```python
from build123d import *

# Parameters (mm, degrees)
SKETCH_1_W          = 210
SKETCH_1_H          = 100
EXTRUDE_1_DEPTH     = 5
FILLET_1_R          = 5
SKETCH_2_R          = 1.5
CUT_EXTRUDE_1_DEPTH = 5
SKETCH_4_R          = 2.25
CUT_EXTRUDE_2_DEPTH = 5
SKETCH_6_R          = 1.5
CUT_EXTRUDE_3_DEPTH = 5


with BuildPart() as part:
    # 草图1 → 凸台-拉伸1 (new body)
    with BuildSketch(Plane(origin=(0, 0, 0), x_dir=(1, 0, 0), z_dir=(0, 1, 0))):
        with Locations((-105, 50)):
            Rectangle(SKETCH_1_W, SKETCH_1_H)
    extrude(amount=EXTRUDE_1_DEPTH)

    # 圆角1
    fillet_1_edges = [part.edges().sort_by_distance(p)[0] for p in [
        (-210, 2.5, -100),
        (0, 2.5, -100),
        (0, 2.5, 0),
        (-210, 2.5, 0),
    ]]
    fillet(fillet_1_edges, radius=FILLET_1_R)

    # 草图2 → 切除-拉伸1 (cut)
    with BuildSketch(Plane(origin=(0, 5, 0), x_dir=(1, 0, 0), z_dir=(0, 1, 0))):
        with Locations(Location((-205, 90, 0), (0, 0, 270))):
            Circle(SKETCH_2_R)
        with Locations(Location((-205, 10, 0), (0, 0, 270))):
            Circle(SKETCH_2_R)
        with Locations(Location((-5, 10, 0), (0, 0, 270))):
            Circle(SKETCH_2_R)
        with Locations(Location((-5, 90, 0), (0, 0, 270))):
            Circle(SKETCH_2_R)
    extrude(amount=-CUT_EXTRUDE_1_DEPTH, mode=Mode.SUBTRACT)

    # 草图4 → 切除-拉伸2 (cut)
    with BuildSketch(Plane.XZ):
        with Locations(Location((-119.1, -45, 0), (0, 0, 270))):
            Circle(SKETCH_4_R)
        with Locations(Location((-119.1, -55, 0), (0, 0, 90))):
            Circle(SKETCH_4_R)
        with Locations(Location((-71.1, -55, 0), (0, 0, 270))):
            Circle(SKETCH_4_R)
        with Locations(Location((-71.1, -45, 0), (0, 0, 90))):
            Circle(SKETCH_4_R)
        Polygon((-115.1, -60), (-75.1, -60), (-75.1, -51), (-71.1, -51), (-71.1, -49), (-75.1, -49), (-75.1, -40), (-115.1, -40), (-115.1, -49), (-119.1, -49), (-119.1, -51), (-115.1, -51), align=None)
    extrude(amount=-CUT_EXTRUDE_2_DEPTH, mode=Mode.SUBTRACT)

    # 草图6 → 切除-拉伸3 (cut)
    with BuildSketch(Plane.XZ):
        with Locations(Location((-40, -41, 0), (0, 0, 270))):
            Circle(SKETCH_6_R)
        with Locations(Location((-40, -59, 0), (0, 0, 270))):
            Circle(SKETCH_6_R)
        with Locations(Location((-170, -59, 0), (0, 0, 90))):
            Circle(SKETCH_6_R)
        with Locations(Location((-170, -41, 0), (0, 0, 90))):
            Circle(SKETCH_6_R)
        with Locations(Location((-185.5, -87, 0), (0, 0, 270))):
            Circle(SKETCH_6_R)
        with Locations(Location((-185.5, -61, 0), (0, 0, 270))):
            Circle(SKETCH_6_R)
        with Locations(Location((-154.5, -87, 0), (0, 0, 90))):
            Circle(SKETCH_6_R)
        with Locations(Location((-154.5, -61, 0), (0, 0, 90))):
            Circle(SKETCH_6_R)
        with Locations(Location((-55.5, -87, 0), (0, 0, 270))):
            Circle(SKETCH_6_R)
        with Locations(Location((-24.5, -87, 0), (0, 0, 90))):
            Circle(SKETCH_6_R)
        with Locations(Location((-55.5, -61, 0), (0, 0, 270))):
            Circle(SKETCH_6_R)
        with Locations(Location((-24.5, -61, 0), (0, 0, 90))):
            Circle(SKETCH_6_R)
    extrude(amount=-CUT_EXTRUDE_3_DEPTH, mode=Mode.SUBTRACT)


solid = part.part
```
CAD build for the part. Positions are in the model's coordinates, mm. A direction names the side the tool comes from. Coordinates: 2 decimals unless noted, no trailing zeros. Write each loop counter-clockwise with the first axis right and the second up, starting at its lowest first coordinate (ties: lowest second). Pieces come first, ordered by that corner, then holes. Notation, with made-up numbers: (-36.5, -30.75) -> (-5.5, -30.75) arc R31 ccw to (-5.5, 2.25) -> close; hole circle Ø4 at (47, 69). An arc over 180 degrees is marked (long way). Return JSON: item names as keys, results as strings. Group by question number.
Q1. Cut at C-C, the plane y = 2.8. State how many separate pieces and enclosed holes the cut face has, then the cut area to 3 significant figures.
Q2. Pull direction Z, two halves, no side cores. Call faces 1 (the face through (-121.296, 2.465, -44.512)), 2 (the face through (-71.001, 2.465, -52.752)), 3 (the face through (-106, 0, -62)), 4 (the face through (-209, 3, -2)): released by +Z, released by -Z, zero draft, split by the parting line, or undercut.
Q3. Cut at A-A, the plane x = -106. Give the cut face in (y, z), then the cut area to 3 significant figures.
Q4. Which spindle directions (+Z, -Z, +X, -X, +Y, -Y) get a long thin tool onto all of the face, cutting with end or side? Do faces 5 (the face through (-106, 2, 0)), 6 (the face through (-117, 2, -51)). Say none if no direction does.
Q5. Drill centre lines: line 1 (X direction, y = 3.05, z = -61); line 2 (X direction, y = 1.75, z = -50.5); line 3 (X direction, y = 0.4, z = -40.5). Where is each one in solid material? Low to high.
Q6. Cut at B-B, the plane z = -45. Give the cut face in (x, y), then the cut area to 3 significant figures.
Returned:
{
 "1": {"separate pieces": "1", "enclosed holes": "21", "area": "20,000 mm2"},
 "2": {"face 1": "undercut", "face 2": "undercut", "face 3": "zero draft", "face 4": "released by +Z"},
 "3": {"outline": "(0, -100) -> (5, -100) -> (5, -60) -> (0, -60) -> close; (0, -40) -> (5, -40) -> (5, 0) -> (0, 0) -> close", "area": "400 mm2"},
 "4": {"face 5": "+Z, +X, -X, +Y, -Y", "face 6": "+Y, -Y"},
 "5": {"line 1": "x = -210 to -187, -184 to -156, -153 to -57, -54 to -26, -23 to 0", "line 2": "x = -210 to -119.1, -71.1 to 0", "line 3": "x = -210 to -171.41, -168.59 to -115.1, -75.1 to -41.41, -38.59 to 0"},
 "6": {"outline": "(-210, 0) -> (-121.35, 0) -> (-121.35, 5) -> (-210, 5) -> close; (-116.85, 0) -> (-115.1, 0) -> (-115.1, 5) -> (-116.85, 5) -> close; (-75.1, 0) -> (-73.35, 0) -> (-73.35, 5) -> (-75.1, 5) -> close; (-68.85, 0) -> (0, 0) -> (0, 5) -> (-68.85, 5) -> close", "area": "805 mm2"}
}
